Autodesk Inventor part; units mm, degrees
ref_plane "YZ Plane" through (0, 0, 0) normal (1, 0, 0) x (0, 1, 0)
ref_plane "XZ Plane" through (0, 0, 0) normal (0, 1, 0) x (-1, 0, 0)
ref_plane "XY Plane" through (0, 0, 0) normal (0, 0, 1) x (1, 0, 0)
sketch "Sketch1" plane through (0, 0, 0) normal (0, 1, 0) x (-1, 0, 0)
  circle A0 centre (0, 0) radius 28.575
  dimension "d0" = 57.15
extrude "Extrusion1" add sketch "Sketch1" along normal blind 0.7937
sketch "Sketch2" plane through (0, 0.7937, 0) normal (0, 1, 0) x (1, 0, 0)
  line L0 (0, 0) -> (-28.575, 0) construction
  circle A0 centre (0, 0) radius 28.575
  line L1 (-6.35, 0) -> (-3.175, 5.4993)
  line L2 (-3.175, 5.4993) -> (3.175, 5.4993)
  line L3 (3.175, 5.4993) -> (6.35, 0)
  line L4 (6.35, 0) -> (3.175, -5.4993)
  line L5 (3.175, -5.4993) -> (-3.175, -5.4993)
  line L6 (-3.175, -5.4993) -> (-6.35, 0)
  circle A1 centre (0, 0) radius 23.8125
  circle A2 centre (0, 0) radius 24.6063
  circle A3 centre (0, 0) radius 27.7812
  circle A4 centre (0, 0) radius 7.493
  circle A5 centre (0, 0) radius 12.7 construction
  circle A6 centre (-12.7, 0) radius 1.7526
  circle A7 centre (-6.35, -10.9985) radius 1.7526
  circle A8 centre (6.35, -10.9985) radius 1.7526
  circle A9 centre (12.7, 0) radius 1.7526
  circle A10 centre (6.35, 10.9985) radius 1.7526
  circle A11 centre (-6.35, 10.9985) radius 1.7526
  dimension "d18" = 25.4
  dimension "d3" = 6.35
  dimension "d4" = 47.625
  dimension "d5" = 0.7937
  dimension "d6" = 0.7937
  dimension "d15" = 14.986
  dimension "d19" = 3.5052
  dimension "d22" = 360
extrude "Extrusion2" add sketch "Sketch2" along normal blind 8.89 contours L1 L2 L3 L4 L5 L6 | A2
fillet "Fillet1" radius 0.508 6 edges at (6.35, 5.2387, 0) (3.175, 5.2387, -5.4993) (-3.175, 5.2387, -5.4993) (-6.35, 5.2387, 0) (-3.175, 5.2387, 5.4993) (3.175, 5.2387, 5.4993)
extrude "Extrusion3" add sketch "Sketch2" along normal blind 12.7 contours A0
chamfer "Chamfer1" distance 0.7937 angle 45 1 edges at (-23.8125, 0.7937, 0)
extrude "Extrusion4" add sketch "Sketch2" along normal blind 1.27 contours L1 L2 L3 L4 L5 L6 | A4
extrude "Extrusion5" cut sketch "Sketch2" against normal through all contours A6 | A7 | A8 | A9 | A10 | A11
properties part number "Wheel V2 Mold"
The model under review builds one solid part; all positions refer to its coordinate system, in mm. A direction names the side the tool comes from. Round coordinates to 2 decimals unless told otherwise and drop trailing zeros. Loops run counter-clockwise (first coordinate to the right, second up) from the corner with the lowest first, then second, coordinate; pieces in that order, holes last.
1) Clearance check with flat-ended pins moving along their axes: P1, Ø4.5, axis at x = -12.7, z = 0, coming from the +Y side; P2, Ø6.5, axis at x = 0, y = 6.5, coming from the +Z side (3 decimals); P3, Ø3, axis at x = -19.5, z = -12, coming from the -Y side; P4, Ø3, axis at y = 2.5, z = 14, coming from the -X side. State where each tip first meets the part, or that it passes through.
Values follow:
P1: stops at y = 0.79
P2: stops at z = 28.575
P3: stops at y = 0
P4: stops at x = -25.7
2) Tool access review of faces 1 (the face through (-3.203, 5.176, 24.397)), 2 (the face through (-14.45, 0.4, -0.08)): name each direction out of +Z, -Z, +X, -X, +Y, -Y from which nothing blocks a thin tool from reaching the whole face with its end or side.
Values follow:
face 1: +Y
face 2: +Y, -Y
3) Wall thickness on line 1 along X through (y, z) = (4, 0) (1 decimal); line 2 along X through (y, z) = (0.45, 0) (3 decimals); line 3 along Z through (x, y) = (0, 7.75) (1 decimal): over which ranges is each line inside the solid? List them lowest first.
Values follow:
line 1: x = -28.6 to -27.8, -24.6 to -23.8, -6.3 to 6.3, 23.8 to 24.6, 27.8 to 28.6
line 2: x = -28.575 to -14.453, -10.947 to 10.947, 14.453 to 28.575
line 3: z = -28.6 to -27.8, -24.6 to -23.8, -5.5 to 5.5, 23.8 to 24.6, 27.8 to 28.6
4) Consider section C-C on y = 12.25. State the section outline as (x, z) points (3 decimals), then the cut area to 3 significant figures.
Values follow:
outline: circle Ø57.15 at (0, 0); hole circle Ø55.562 at (0, 0)
area: 141 mm2
5) Consider section A-A on y = 4.75. Give the number of separate pieces and of enclosed holes in the cut face, then the cut area to 3 significant figures.
Values follow:
separate pieces: 3
enclosed holes: 2
area: 366 mm2
